Could you check a few things on this model? Use its own coordinates, in mm. Coordinates: 2 decimals unless noted, no trailing zeros. Loops run counter-clockwise (first coordinate to the right, second up) from the corner with the lowest first, then second, coordinate; pieces in that order, holes last. Notation, with made-up numbers: (85.25, 16) - (141.25, 16) arc R6 ccw to (141.25, 20) - close; hole circle Ø5 at (-11.75, 55.5). An arc over 180 degrees is marked (long way). Use CSV: the item, a comma, the result in double quotes.
Autodesk Inventor part; units mm, degrees
ref_plane "Work Plane2" through (170.5249, -159.3871, 0) normal (0.9993154, -0.0369972, 0) x (0.0369972, 0.9993154, 0)
ref_plane "YZ Plane" through (0, 0, 0) normal (1, 0, 0) x (0, 1, 0)
ref_plane "XZ Plane" through (0, 0, 0) normal (0, 1, 0) x (-1, 0, 0)
sketch "Sketch1" plane through (0, 0, 0) normal (0, 0, 1) x (1, 0, 0)
  circle A0 centre (0, 0) radius 6.05
surface extrude "ExtrusionSrf1" sketch "Sketch1" along normal mid plane 6 shown yes curves A0
sketch "Sketch2" plane through (0, 0, 0) normal (0, 0, 1) x (1, 0, 0)
  circle A0 centre (324.834, -10.3853) radius 6.05
  point P0 (0, 0)
surface extrude "ExtrusionSrf2" sketch "Sketch2" along normal mid plane 6 shown yes curves A0
sketch "Sketch3" plane through (0, 0, 0) normal (0, 0, 1) x (1, 0, 0)
  circle A0 centre (-9.3308, -291.8509) radius 6.11
  point P0 (0, 0)
surface extrude "ExtrusionSrf3" sketch "Sketch3" along normal blind 6 shown yes curves A0
sketch "Sketch4" plane through (0, 0, 0) normal (0, 0, 1) x (1, 0, 0)
  circle A0 centre (7.3217, -169.3662) radius 5.735
  point P0 (0, 0)
surface extrude "ExtrusionSrf4" sketch "Sketch4" along normal mid plane 6 shown yes curves A0
sketch "Sketch5" plane through (0, 0, 0) normal (0, 0, 1) x (1, 0, 0)
  circle A0 centre (319.839, -166.6212) radius 6.05
  point P0 (0, 0)
surface extrude "ExtrusionSrf5" sketch "Sketch5" along normal mid plane 6 shown yes curves A0
sketch "Sketch6" plane through (0, 0, 0) normal (0, 0, 1) x (1, 0, 0)
  circle A0 centre (135.3864, -162.1898) radius 3
  point P0 (0, 0)
surface extrude "ExtrusionSrf6" sketch "Sketch6" along normal mid plane 6 shown yes curves A0
sketch "Sketch7" plane through (0, 0, 0) normal (0, 0, 1) x (1, 0, 0)
  circle A0 centre (154.3767, -162.797) radius 3
  point P0 (0, 0)
surface extrude "ExtrusionSrf7" sketch "Sketch7" along normal mid plane 6 shown yes curves A0
sketch "Sketch8" plane through (0, 0, 0) normal (0, 0, 1) x (1, 0, 0)
  circle A0 centre (0, 0) radius 6.05
  circle A1 centre (7.3217, -169.3662) radius 5.735
  circle A2 centre (-9.3308, -291.8509) radius 6.11
  circle A3 centre (135.3864, -162.1898) radius 3
  circle A4 centre (154.3767, -162.797) radius 3
  circle A5 centre (319.839, -166.6212) radius 6.05
  circle A6 centre (324.834, -10.3853) radius 6.05
  arc A7 (0.2015, 6.3018) -> (-6.3017, 0.2028) centre (0, 0) ccw
  arc A8 (-15.6925, -291.6462) -> (-2.969, -292.0543) centre (-9.3308, -291.8509) ccw
  arc A9 (7.4805, -163.0032) -> (0.9599, -169.1628) centre (7.3217, -169.3662) ccw
  arc A10 (135.2865, -166.1936) -> (135.4863, -158.1861) centre (135.3864, -162.1898) ccw
  arc A11 (331.1358, -10.5868) -> (325.0355, -4.0835) centre (324.834, -10.3853) ccw
  arc A12 (154.5249, -158.7947) -> (154.2285, -166.7992) centre (154.3767, -162.797) ccw
  arc A13 (319.6057, -172.9219) -> (326.1408, -166.8227) centre (319.839, -166.6212) ccw
  line L0 (-15.6925, -291.6462) -> (-6.3017, 0.2028)
  line L1 (0.2015, 6.3018) -> (325.0355, -4.0835)
  line L2 (-2.969, -292.0543) -> (0.9599, -169.1628)
  line L3 (7.4805, -163.0032) -> (135.2865, -166.1936)
  line L4 (331.1358, -10.5868) -> (326.1408, -166.8227)
  line L5 (119.4863, -157.7867) -> (135.4863, -158.1861)
  line L6 (154.2285, -166.7992) -> (319.6057, -172.9219)
  line L7 (154.5249, -158.7947) -> (170.5249, -159.3871)
  dimension "d14" = 0.255
  dimension "d15" = 0.255
  dimension "d16" = 0.255
  dimension "d17" = 0.63
  dimension "d19" = 0.255
  dimension "d22" = 1.005
  dimension "d23" = 1.005
  dimension "d34" = 16
  dimension "d35" = 16
ref_plane "Work Plane2" through (170.5249, -159.3871, 0) normal (0.9993154, -0.0369972, 0) x (0.0369972, 0.9993154, 0)
sketch "Sketch10" plane through (170.5249, -159.3871, 0) normal (0.9993154, -0.0369972, 0) x (0.0369972, 0.9993154, 0)
  line L0 (0.63, 3) -> (-0.255, 3)
  line L1 (-0.255, 3) -> (-0.255, -3)
  line L2 (-0.255, -3) -> (0.63, -3)
  line L3 (0.63, -3) -> (0.63, 3)
  line L4 (0.63, 0) -> (-0.255, 0) construction
  point P0 (152.969, 0)
  point P1 (0, 0)
  dimension "d29" = 6
  dimension "d30" = 0.63
  dimension "d31" = 0.255
sweep "Sweep2" add profiles "Sketch10" path "Sketch8" path curves L7 A12 L6 A13 L4 A11 L1 A7 L0 A8 L2 A9 L3 A10 L5
equation "\"d14\" = inside"
equation "\"d15\" = inside"
equation "\"d16\" = inside"
equation "\"d17\" = backside"
equation "\"d19\" = inside"
equation "\"inside\" = 0.255"
equation "\"backside\" = 0.63"
properties part number "Belt 1" material "Rubber"
(1) Suppose I cut it at B-B (y = -135.5). Write out the boundary of the cut face in (x, z).
Computed:
outline,"(-11.3, -3) - (-10.41, -3) - (-10.41, 3) - (-11.3, 3) - close; (326.89, -3) - (327.77, -3) - (327.77, 3) - (326.89, 3) - close"
(2) Suppose I cut it at A-A (x = 100). Write out the boundary of the cut face in (y, z).
Computed:
outline,"(-165.94, -3) - (-165.06, -3) - (-165.06, 3) - (-165.94, 3) - close; (2.86, -3) - (3.74, -3) - (3.74, 3) - (2.86, 3) - close"
(3) Will these pins go through, and if not, where does the flat tip stop? pin 1 (3 mm diameter, centred on x = 296, z = -2, fed in from +Y); pin 2 (1.5 mm diameter, centred on x = 164.5, z = 2, fed in from -Y); pin 3 (1 mm diameter, centred on y = -105, z = -1.5, fed in from +X).
Computed:
pin 1,"stops at y = -2.48"
pin 2,"stops at y = -167.84"
pin 3,"stops at x = 328.76"
(4) Please list where these lines run through material, in increasing order: line 1 (X direction, y = -52, z = 1.3); line 2 (Y direction, x = 225, z = -2.4); line 3 (X direction, y = -122.5, z = -0.9).
Computed:
line 1,"x = -8.61 to -7.73, 329.56 to 330.44"
line 2,"y = -170.05 to -169.16, -1.14 to -0.25"
line 3,"x = -10.88 to -9.99, 327.3 to 328.19"
